from build123d import *

# Parameters (mm, degrees)
SKETCH_1_W          = 220
SKETCH_1_H          = 130
EXTRUDE_1_DEPTH     = 110
SKETCH_2_W          = 190
SKETCH_2_H          = 110
CUT_EXTRUDE_1_DEPTH = 169.597153001
ST9_5_1_D           = 10
SKETCH_5_W          = 50
SKETCH_5_H          = 20
EXTRUDE_2_DEPTH     = 40
HOLE_WIZARD_M16_1_D = 14
FILLET_1_R          = 10


with BuildPart() as part:
    # 草图1 → 凸台-拉伸1 (new body)
    with BuildSketch(Plane.XY):
        Rectangle(SKETCH_1_W, SKETCH_1_H)
    extrude(amount=EXTRUDE_1_DEPTH)

    # 草图2 → 切除-拉伸1 (cut, through all)
    with BuildSketch(Plane.XY.offset(110)):
        with Locations((0, -10)):
            Rectangle(SKETCH_2_W, SKETCH_2_H)
    extrude(amount=-CUT_EXTRUDE_1_DEPTH, mode=Mode.SUBTRACT)

    # ST9.5 间隙孔1 (through all)
    with Locations(Plane.ZY.offset(110)):
        with Locations((23, 27), (85, 27), (85, -55), (23, -55)):
            Hole(ST9_5_1_D / 2)

    # 草图5 → 凸台-拉伸2 (add)
    with BuildSketch(Plane(origin=(0, 0, 0), x_dir=(-1, 0, 0), z_dir=(0, 0, -1))):
        with Locations((0, 55)):
            Rectangle(SKETCH_5_W, SKETCH_5_H)
    extrude(amount=EXTRUDE_2_DEPTH)

    # M16 螺纹孔1 (through all)
    with Locations(Plane(origin=(0, 65, 0), x_dir=(1, 0, 0), z_dir=(0, 1, 0))):
        with Locations((0, 30)):
            Hole(HOLE_WIZARD_M16_1_D / 2)

    # 圆角1
    fillet_1_edges = [part.edges().sort_by_distance(p)[0] for p in [
        (25, 55, -40),
        (-25, 55, -40),
    ]]
    fillet(fillet_1_edges, radius=FILLET_1_R)


solid = part.part
Can you work these out from the model? Positions are in its coordinate system, mm. A direction names the side the tool comes from. Coordinates: 2 decimals unless noted, no trailing zeros. Write each loop counter-clockwise with the first axis right and the second up, starting at its lowest first coordinate (ties: lowest second). Pieces come first, ordered by that corner, then holes. Notation, with made-up numbers: (53.5, 38.25) - (64.5, 38.25) arc R26 cw to (64.5, 72.25) - close; hole circle Ø1 at (52.25, 43). An arc over 180 degrees is marked (long way). Return JSON: item names as keys, results as strings. Group by question number.
Item 1: We'd pull the mould along X, two halves only. Please class faces 1 (the face through (-25, 55, -15)), 2 (the face through (-95, -11, 56)), 3 (the face through (-2, 65, 51)): pulls with the +X half, pulls with the -X half, needs draft (parallel to the pull), parting line crosses it, or undercut.
Item 2: I'm going to push flat-ended pins straight in: pin 1 Ø10 at (y, z) = (56, -13.5) entering from -X; pin 2 Ø1.5 at (x, z) = (82, 4.5) entering from -Y; pin 3 Ø22 at (y, z) = (50, -13) entering from +X. Where does each tip first touch, or does it pass through?
Item 3: If we section it at B-B (y = 27): Write out the boundary of the cut face in (x, z).
Item 4: Please list where these lines run through material, in increasing order: probe 1 along Y at (x, z) = (-104.5, 85); probe 2 along X at (y, z) = (-12, 3); probe 3 along X at (y, z) = (52.5, -30).
Item 5: If we section it at C-C (z = 85): Write out the boundary of the cut face in (x, y), then the cut area to 3 significant figures.
Item 6: If we section it at A-A (x = 0): Write out the boundary of the cut face in (y, z).
Item 7: Which directions (+Z, -Z, +X, -X, +Y, -Y) give clear straight access to the entire face, cutting with the end or side of a thin tool? Please do faces 4 (the face through (96, 29, 0)), 5 (the face through (110, -1, 54)), 6 (the face through (95, -11, 56)).
Item 8: If we section it at D-D (y = -31.5): Write out the boundary of the cut face in (x, z), then the cut area to 3 significant figures.
Return value:
{
 "1": {"face 1": "pulls with the -X half", "face 2": "undercut", "face 3": "needs draft"},
 "2": {"pin 1": "stops at x = -25", "pin 2": "stops at y = 45", "pin 3": "stops at x = 25"},
 "3": {"outline": "(-110, 0) - (-95, 0) - (-95, 18) - (-110, 18) - close; (-110, 28) - (-95, 28) - (-95, 80) - (-110, 80) - close; (-110, 90) - (-95, 90) - (-95, 110) - (-110, 110) - close; (95, 0) - (110, 0) - (110, 18) - (95, 18) - close; (95, 28) - (110, 28) - (110, 80) - (95, 80) - close; (95, 90) - (110, 90) - (110, 110) - (95, 110) - close"},
 "4": {"probe 1": "y = -65 to -60, -50 to 22, 32 to 65", "probe 2": "x = -110 to -95, 95 to 110", "probe 3": "x = -25 to -7, 7 to 25"},
 "5": {"outline": "(-110, -65) - (-95, -65) - (-95, -60) - (-110, -60) - close; (-110, -50) - (-95, -50) - (-95, 22) - (-110, 22) - close; (-110, 32) - (-95, 32) - (-95, 45) - (95, 45) - (95, 32) - (110, 32) - (110, 65) - (-110, 65) - close; (95, -65) - (110, -65) - (110, -60) - (95, -60) - close; (95, -50) - (110, -50) - (110, 22) - (95, 22) - close", "area": "7,100 mm^2"},
 "6": {"outline": "(45, -40) - (65, -40) - (65, -37) - (45, -37) - close; (45, -23) - (65, -23) - (65, 110) - (45, 110) - close"},
 "7": {"face 4": "-Z, +X, +Y, -Y", "face 5": "+Z, -Z, +X, +Y, -Y", "face 6": "+Z, -Z, -Y"},
 "8": {"outline": "(-110, 0) - (-95, 0) - (-95, 110) - (-110, 110) - close; (95, 0) - (110, 0) - (110, 110) - (95, 110) - close", "area": "3,300 mm^2"}
}
